For this review, take the finished solid that the model builds, in its own axes (mm). Give positions to 0.01 mm unless a question says otherwise; leave off trailing zeros.
```python
from build123d import *

# Parameters (mm, degrees)
SKETCH2_R           = 3
SKETCH2_R_2         = 31
BOSS_EXTRUDE1_DEPTH = 8
CHAMFER1_SIZE       = 8


with BuildPart() as part:
    # Sketch2 → Boss-Extrude1 (new body)
    with BuildSketch(Plane.XY):
        with BuildLine():
            ThreePointArc((50.792573497, 18.265840665), (51.961524227, 30), (41.214968786, 34.85473864))
            ThreePointArc((41.214968786, 34.85473864), (36.65999643, 34.997336465), (32.641290086, 37.146314508))
            ThreePointArc((32.641290086, 37.146314508), (24.725, 42.824956217), (15.849006977, 46.841343681))
            ThreePointArc((15.849006977, 46.841343681), (11.978584229, 49.247156444), (9.577604711, 53.120579305))
            ThreePointArc((9.577604711, 53.120579305), (0, 60), (-9.577604711, 53.120579305))
            ThreePointArc((-9.577604711, 53.120579305), (-11.978584229, 49.247156444), (-15.849006977, 46.841343681))
            ThreePointArc((-15.849006977, 46.841343681), (-24.725, 42.824956217), (-32.641290086, 37.146314508))
            ThreePointArc((-32.641290086, 37.146314508), (-36.65999643, 34.997336465), (-41.214968786, 34.85473864))
            ThreePointArc((-41.214968786, 34.85473864), (-51.961524227, 30), (-50.792573497, 18.265840665))
            ThreePointArc((-50.792573497, 18.265840665), (-48.638580659, 14.249819979), (-48.490297064, 9.695029173))
            ThreePointArc((-48.490297064, 9.695029173), (-49.45, 0), (-48.490297064, -9.695029173))
            ThreePointArc((-48.490297064, -9.695029173), (-48.638580659, -14.249819979), (-50.792573497, -18.265840665))
            ThreePointArc((-50.792573497, -18.265840665), (-51.961524227, -30), (-41.214968786, -34.85473864))
            ThreePointArc((-41.214968786, -34.85473864), (-36.65999643, -34.997336465), (-32.641290086, -37.146314508))
            ThreePointArc((-32.641290086, -37.146314508), (-24.725, -42.824956217), (-15.849006977, -46.841343681))
            ThreePointArc((-15.849006977, -46.841343681), (-11.978584229, -49.247156444), (-9.577604711, -53.120579305))
            ThreePointArc((-9.577604711, -53.120579305), (0, -60), (9.577604711, -53.120579305))
            ThreePointArc((9.577604711, -53.120579305), (11.978584229, -49.247156444), (15.849006977, -46.841343681))
            ThreePointArc((15.849006977, -46.841343681), (24.725, -42.824956217), (32.641290086, -37.146314508))
            ThreePointArc((32.641290086, -37.146314508), (36.65999643, -34.997336465), (41.214968786, -34.85473864))
            ThreePointArc((41.214968786, -34.85473864), (51.961524227, -30), (50.792573497, -18.265840665))
            ThreePointArc((50.792573497, -18.265840665), (48.638580659, -14.249819979), (48.490297064, -9.695029173))
            ThreePointArc((48.490297064, -9.695029173), (49.45, 0), (48.490297064, 9.695029173))
            ThreePointArc((48.490297064, 9.695029173), (48.638580659, 14.249819979), (50.792573497, 18.265840665))
        make_face()
        with Locations((45.899346401, 26.5)):
            Circle(SKETCH2_R, mode=Mode.SUBTRACT)
        with Locations((0, 53)):
            Circle(SKETCH2_R, mode=Mode.SUBTRACT)
        Circle(SKETCH2_R_2, mode=Mode.SUBTRACT)
        with Locations((45.899346401, -26.5)):
            Circle(SKETCH2_R, mode=Mode.SUBTRACT)
        with Locations((0, -53)):
            Circle(SKETCH2_R, mode=Mode.SUBTRACT)
        with Locations((-45.899346401, 26.5)):
            Circle(SKETCH2_R, mode=Mode.SUBTRACT)
        with Locations((-45.899346401, -26.5)):
            Circle(SKETCH2_R, mode=Mode.SUBTRACT)
    extrude(amount=BOSS_EXTRUDE1_DEPTH)

    # Chamfer1
    chamfer1_edges = [part.edges().sort_by_distance(p)[0] for p in [
        (-31, 0, 8),
    ]]
    chamfer(chamfer1_edges, length=CHAMFER1_SIZE - 0.0001)  # a hair under: the kernel refuses the full size


solid = part.part
```
Item 1: Clearance check with a flat-ended pin moving along its axis: pin 1 Ø1.5 at (x, z) = (3.5, 3) entering from +Y. State where the tip first meets the part, or that it passes through.
Answer:
pin 1: stops at y = 59.62
Item 2: Take a section at B-B on x = 0. State how many separate pieces and enclosed holes the cut face has, and give its area (3 significant figures).
Answer:
separate pieces: 4
enclosed holes: 0
area: 304 mm2
Item 3: The part is to be moulded in two halves that separate along X. For faces 1 (the cylindrical face through (48.622, 14.188, 3.944)), 2 (the cylindrical face through (-48.655, 14.312, 3.944)), 3 (the cylindrical face through (36.598, -35.014, 3.944)), say which applies: released by +X, released by -X, zero draft, split by the parting line, or undercut.
Answer:
face 1: released by +X
face 2: released by -X
face 3: undercut
Item 4: For L1, parallel to Y at x = -39, z = 2; L2, parallel to Y at x = -42.5, z = 3.5; L3, parallel to X at y = -15, z = 1.25, list the stretches that pass through material, from the lowest coordinate up.
Answer:
L1: y = -34.66 to 34.66
L2: y = -35.03 to 35.03
L3: x = -48.87 to -28.55, 28.55 to 48.87
